from build123d import *

# Parameters (mm, degrees)
BOSS_EXTRUDE1_DEPTH = 30
SKETCH2_R           = 12.5
CUT_EXTRUDE1_DEPTH  = 5
SKETCH3_R           = 3
SKETCH3_R_2         = 1.5
CUT_EXTRUDE3_DEPTH  = 10
SKETCH5_W           = 15
SKETCH5_H           = 32
CUT_EXTRUDE4_DEPTH  = 31
SKETCH6_R           = 1.5
SKETCH6_W           = 15
SKETCH6_H           = 22
CUT_EXTRUDE5_DEPTH  = 175.419035658
FILLET2_R           = 10
CHAMFER2_SIZE       = 2
SKETCH7_W           = 20
SKETCH7_H           = 90
CUT_EXTRUDE6_DEPTH  = 173.690474549
FILLET3_R           = 10
FILLET4_R           = 1
FILLET5_R           = 3


with BuildPart() as part:
    # Sketch1 → Boss-Extrude1 (new body)
    with BuildSketch(Plane.XY):
        with BuildLine():
            Line((19, 150), (19, 0))
            ThreePointArc((19, 0), (0, -19), (-19, 0))
            Line((-19, 0), (-19, 150))
            Line((-19, 150), (-19, 169))
            Line((-19, 169), (19, 169))
            Line((19, 169), (19, 150))
        make_face()
    extrude(amount=BOSS_EXTRUDE1_DEPTH)

    # Sketch2 → Cut-Extrude1 (cut)
    with BuildSketch(Plane.XY.offset(30)):
        Circle(SKETCH2_R)
    extrude(amount=-CUT_EXTRUDE1_DEPTH, mode=Mode.SUBTRACT)

    # Sketch3 → Cut-Extrude3 (cut)
    with BuildSketch(Plane.XY.offset(25)):
        Circle(SKETCH3_R)
        with Locations((0, 7.5)):
            Circle(SKETCH3_R_2)
        with Locations((7.5, 0)):
            Circle(SKETCH3_R_2)
        with Locations((0, -7.5)):
            Circle(SKETCH3_R_2)
        with Locations((-7.5, 0)):
            Circle(SKETCH3_R_2)
    extrude(amount=-CUT_EXTRUDE3_DEPTH, mode=Mode.SUBTRACT)

    # Sketch5 → Cut-Extrude4 (cut)
    with BuildSketch(Plane.ZY.offset(19)):
        with Locations((15, 139)):
            Rectangle(SKETCH5_W, SKETCH5_H)
    extrude(amount=-CUT_EXTRUDE4_DEPTH, mode=Mode.SUBTRACT)

    # Sketch6 → Cut-Extrude5 (cut, through all)
    with BuildSketch(Plane.ZY.offset(-12)):
        with Locations((12, 152.5)):
            Circle(SKETCH6_R)
        with Locations(Location((18, 152.5, 0), (0, 0, 180))):
            Circle(SKETCH6_R)
        with Locations((18, 125.5)):
            Circle(SKETCH6_R)
        with Locations(Location((12, 125.5, 0), (0, 0, 180))):
            Circle(SKETCH6_R)
        with Locations((15, 139)):
            Rectangle(SKETCH6_W, SKETCH6_H)
    extrude(amount=-CUT_EXTRUDE5_DEPTH, mode=Mode.SUBTRACT)

    # Fillet2
    fillet2_edges = [part.edges().sort_by_distance(p)[0] for p in [
        (-19, 169, 15),
        (19, 169, 15),
    ]]
    fillet(fillet2_edges, radius=FILLET2_R)

    # Chamfer2
    chamfer2_edges = [part.edges().sort_by_distance(p)[0] for p in [
        (16.071067812, 166.071067812, 30),
        (0, -19, 30),
        (19, 79.5, 30),
        (19, 79.5, 0),
        (0, -19, 0),
        (0, 169, 0),
        (0, 169, 30),
        (-19, 79.5, 0),
        (-16.071067812, 166.071067812, 0),
        (16.071067812, 166.071067812, 0),
        (-19, 79.5, 30),
        (-16.071067812, 166.071067812, 30),
    ]]
    chamfer(chamfer2_edges, length=CHAMFER2_SIZE)

    # Sketch7 → Cut-Extrude6 (cut, through all)
    with BuildSketch(Plane(origin=(0, 0, 0), x_dir=(-1, 0, 0), z_dir=(0, 0, -1))):
        with Locations((0, 65)):
            Rectangle(SKETCH7_W, SKETCH7_H)
    extrude(amount=-CUT_EXTRUDE6_DEPTH, mode=Mode.SUBTRACT)

    # Fillet3
    fillet3_edges = [part.edges().sort_by_distance(p)[0] for p in [
        (-10, 110, 15),
        (10, 20, 15),
        (-10, 20, 15),
        (10, 110, 15),
    ]]
    fillet(fillet3_edges, radius=FILLET3_R - 0.0001)  # a hair under: the kernel refuses the full size

    # Fillet4
    fillet4_edges = [part.edges().sort_by_distance(p)[0] for p in [
        (-3.5, 155, 22.5),
        (-3.5, 123, 22.5),
        (-3.5, 123, 7.5),
        (-3.5, 155, 7.5),
    ]]
    fillet(fillet4_edges, radius=FILLET4_R)

    # Fillet5
    fillet5_edges = [part.edges().sort_by_distance(p)[0] for p in [
        (-10, 65, 0),
        (-10, 65, 30),
        (10, 65, 0),
        (10, 65, 30),
        (-7.071097101, 107.071097101, 0),
        (-7.071097101, 107.071097101, 30),
        (7.071097101, 22.928902899, 0),
        (7.071097101, 22.928902899, 30),
        (-7.071097101, 22.928902899, 0),
        (-7.071097101, 22.928902899, 30),
        (7.071097101, 107.071097101, 0),
        (7.071097101, 107.071097101, 30),
    ]]
    fillet(fillet5_edges, radius=FILLET5_R)


solid = part.part
Part model, mm, in its own coordinate system. A direction names the side the tool comes from. Give positions to 0.01 mm unless a question says otherwise; leave off trailing zeros. Order: outer loops, then holes, each group sorted by start corner. A loop starts at its lowest first (then second) coordinate and runs counter-clockwise, first axis right, second up. Notation, with made-up numbers: (28.5, 56.5) - (87.5, 56.5) arc R10 cw to (87.5, 74.5) - close; hole circle Ø11 at (-5.75, 56.5). An arc over 180 degrees is marked (long way). One line per question, with ' | ' between items.
1. Drill centre lines: probe 1 along Z at (x, y) = (14.5, 152.5); probe 2 along Y at (x, z) = (0, 21.75); probe 3 along Y at (x, z) = (0, 27.15). Where is each one in solid material? Low to high.
Filled in:
probe 1: 0 to 10.5, 13.5 to 16.5, 19.5 to 30 | probe 2: -19 to -9, -6 to -3, 3 to 6, 9 to 20, 110 to 123.03, 154.97 to 169 | probe 3: -19 to -12.5, 12.5 to 20, 110 to 169
2. Which spindle directions (+Z, -Z, +X, -X, +Y, -Y) get a long thin tool onto all of the face, cutting with end or side? Do faces 1 (the face through (-7.15, 106.99, 15.17)), 2 (the face through (-10.9, 65.49, 0.86)), 3 (the face through (12, 126, 15)), 4 (the face through (10.9, 64.51, 29.14)). Say none if no direction does.
Filled in:
face 1: +Z, -Z | face 2: -Z | face 3: -X | face 4: +Z
3. Band-saw the part on A-A on y = 84. List the corners of the cut face in (x, z), then the cut area to 3 significant figures.
Filled in:
outline: (-19, 2) - (-17, 0) - (-13, 0) arc R3 ccw to (-10, 3) - (-10, 27) arc R3 ccw to (-13, 30) - (-17, 30) - (-19, 28) - close; (10, 3) arc R3 ccw to (13, 0) - (17, 0) - (19, 2) - (19, 28) - (17, 30) - (13, 30) arc R3 ccw to (10, 27) - close | area: 524 mm²
4. Drop flat-ended pins along their axis: P1, Ø1, axis at x = -13.5, z = 23, coming from the -Y side; P2, Ø2.5, axis at x = 7.5, y = 0, coming from the +Z side; P3, Ø6.5, axis at x = 0.5, y = 0.5, coming from the +Z side. Give the stop position or say it passes through.
Filled in:
P1: y = -13.86 | P2: z = 15 | P3: z = 25
5. Pull direction Z, two halves, no side cores. Call faces 5 (the face through (0, -9, 20)), 6 (the face through (0, 139, 22.5)), 7 (the face through (-15.11, 164.97, 0.54)): +Z half, -Z half, draft (parallel to the pull), parting line (faces both ways), or undercut.
Filled in:
face 5: draft | face 6: undercut | face 7: -Z half
